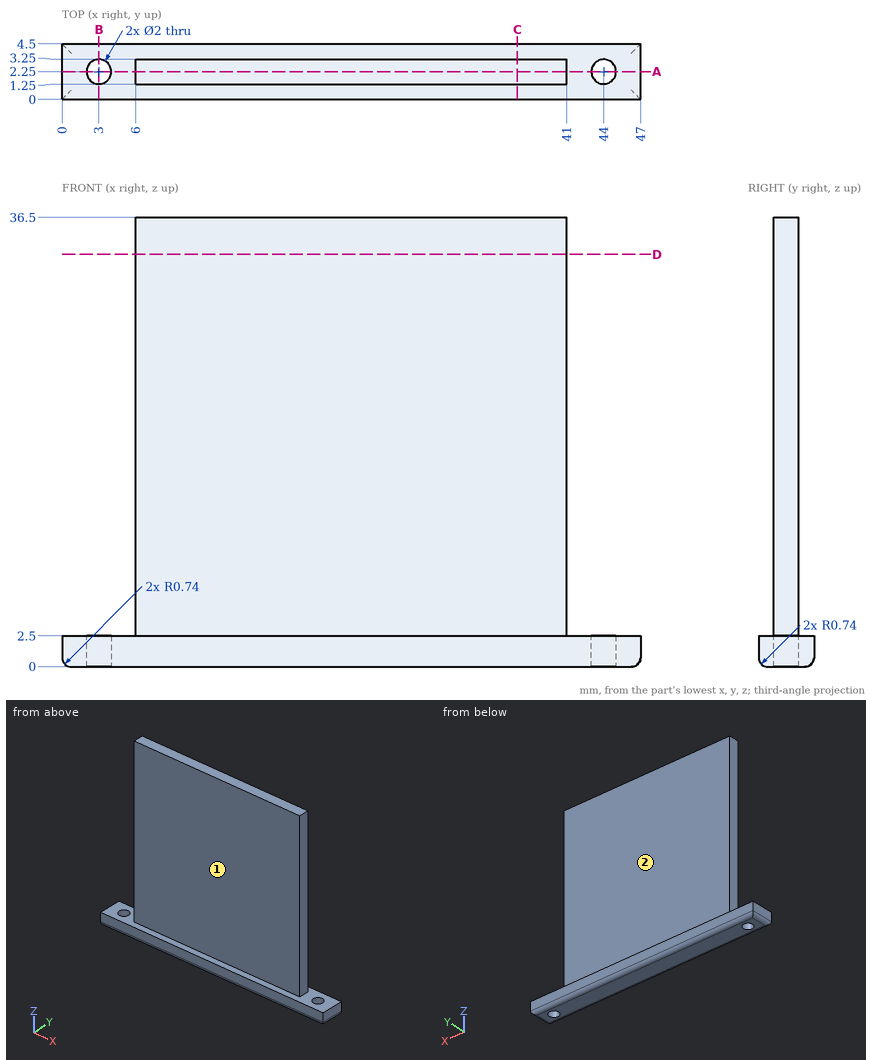
Geometry: see drawing. Coordinates: mm, zero at the bounding-box minimum. A direction names the side the tool comes from. Coordinates: 2 decimals unless noted, no trailing zeros. Order: outer loops, then holes, each group sorted by start corner. A loop starts at its lowest first (then second) coordinate and runs counter-clockwise, first axis right, second up. Notation, with made-up numbers: M 46,15.25 L 101,15.25 A10 ccw 101,29.25 Z; hole C 62,-31 d7. An arc over 180 degrees is marked long. Write each question's results on one line, items separated by ' | '. Start each with the question number.
1) Contact query for flat-ended pins moving along their axis: pin 1 Ø2.5 at (x, y) = (3, 2.25) entering from -Z; pin 2 Ø1.6 at (x, y) = (44, 2.25) entering from +Z; pin 3 Ø0.6 at (y, z) = (2.5, 20) entering from +X; pin 4 Ø17 at (x, z) = (18, 20) entering from -Y. Output: stop coordinate, or through.
2) Access query for the marked faces 1 and 2. Directions: +Z, -Z, +X, -X, +Y, -Y. A direction counts if a zero-diameter tool reaches every point of the face in a straight line with its end or side. Return the directions, or none.
3) Section query C-C (x = 37). Return the cut outline in (y, z).
4) Section query B-B (x = 3). Return the cut outline in (y, z), plus the area to 3 significant figures.
5) Section query D-D (z = 33.5). Return the cut outline in (x, y).
6) Line query: line 1 (Y direction, x = 3, z = 1); line 2 (Z direction, x = 13, y = 1.1); line 3 (Y direction, x = 27, z = 26). Output: solid intervals per line, ascending. Write a range as from..to.
7) Section query A-A (y = 2.25). Return the cut outline in (x, z).
Answers:
1) pin 1: stops at z = 0 | pin 2: passes through | pin 3: stops at x = 41 | pin 4: stops at y = 1.25
2) face 1: +Z, +X, -X, -Y | face 2: +Z, +X, -X, +Y
3) outline: M 0,0.74 A0.74 ccw 0.74,0 L 3.76,0 A0.74 ccw 4.5,0.74 L 4.5,2.5 L 3.25,2.5 L 3.25,36.5 L 1.25,36.5 L 1.25,2.5 L 0,2.5 Z
4) outline: M 0,0.74 A0.74 ccw 0.74,0 L 1.25,0 L 1.25,2.5 L 0,2.5 Z; M 3.25,0 L 3.76,0 A0.74 ccw 4.5,0.74 L 4.5,2.5 L 3.25,2.5 Z | area: 6.01 mm^2
5) outline: M 6,1.25 L 41,1.25 L 41,3.25 L 6,3.25 Z
6) line 1: y = 0..1.25, 3.25..4.5 | line 2: z = 0..2.5 | line 3: y = 1.25..3.25
7) outline: M 0,0.74 A0.74 ccw 0.74,0 L 2,0 L 2,2.5 L 0,2.5 Z; M 4,0 L 43,0 L 43,2.5 L 41,2.5 L 41,36.5 L 6,36.5 L 6,2.5 L 4,2.5 Z; M 45,0 L 46.26,0 A0.74 ccw 47,0.74 L 47,2.5 L 45,2.5 Z
